Could you check a few things on this model? Use its own coordinates, in mm. A direction names the side the tool comes from. Give positions to 0.01 mm unless a question says otherwise; leave off trailing zeros. Loops run counter-clockwise (first coordinate to the right, second up) from the corner with the lowest first, then second, coordinate; pieces in that order, holes last. Notation, with made-up numbers: M -39,51 L -34,51 A27 cw -34,76 Z; hole C 41.25,44 d9. An arc over 180 degrees is marked long. Use a Markdown table: item, result. Add a question column.
1) Suppose I cut it at D-D on x = 8.5. List the corners of the cut face in (y, z) for me, and give its area (3 significant figures).
2) We'd pull the mould along Z, two halves only. Please class faces 3 (the flat face through (0, 0, -92.202)), 4 (the flat face through (0, 0, 0)), 5 (the cylindrical face through (1.323, 10.074, -70.11)): +Z half, -Z half, draft (parallel to the pull), parting line (faces both ways), or undercut.
3) If I drill on line 1 along Z through (x, y) = (7.25, 3.5); line 2 along Y through (x, z) = (-0.25, -9.5); line 3 along X through (y, z) = (2.5, -30.5), over which ranges is the centre line in solid material (lowest first)? Write a range as [from, to].
4) Which directions (+Z, -Z, +X, -X, +Y, -Y) give clear straight access to the entire face, cutting with the end or side of a thin tool? Please do faces 1 (the cylindrical face through (-1.38, -6.2, -29.8)), 2 (the flat face through (0, -7, -79.502)).
5) Suppose I cut it at C-C on z = -50. List the corners of the cut face in (x, y) for me.
6) Suppose I cut it at A-A on y = 0. List the corners of the cut face in (x, z) for me, and give its area (3 significant figures).
7) Will these pins go through, and if not, where does the flat tip stop? pin 1 Ø6 at (x, z) = (4, -66.5) entering from -Y; pin 2 Ø12 at (y, z) = (6, -56) entering from +X; pin 3 Ø8 at (y, z) = (-2.5, -40.5) entering from -X.
```python
from build123d import *

# Parameters (mm, degrees)
SKETCH1_R           = 6.35
BOSS_EXTRUDE1_DEPTH = 92.202
BOSS_EXTRUDE2_START = -12.7
SKETCH2_R           = 10.16
BOSS_EXTRUDE2_DEPTH = 19.05


with BuildPart() as part:
    # Sketch1 → Boss-Extrude1 (new body)
    with BuildSketch(Plane.XY):
        Circle(SKETCH1_R)
    extrude(amount=-BOSS_EXTRUDE1_DEPTH)

    # Sketch2 → Boss-Extrude2 (add)
    with BuildSketch(Plane(origin=(0, 0, -92.202), x_dir=(-1, 0, 0), z_dir=(0, 0, -1)).offset(BOSS_EXTRUDE2_START)):
        Circle(SKETCH2_R)
    extrude(amount=-BOSS_EXTRUDE2_DEPTH)


solid = part.part
```
Answer block:
| question | item | result |
|---|---|---|
| 1 | outline | M -5.57,-79.5 L 5.57,-79.5 L 5.57,-60.45 L -5.57,-60.45 Z |
| 1 | area | 212 mm^2 |
| 2 | face 3 | -Z half |
| 2 | face 4 | +Z half |
| 2 | face 5 | draft |
| 3 | line 1 | z = [-79.5, -60.45] |
| 3 | line 2 | y = [-6.35, 6.35] |
| 3 | line 3 | x = [-5.84, 5.84] |
| 4 | face 1 | +Z |
| 4 | face 2 | -Z |
| 5 | outline | C 0,0 d12.7 |
| 6 | outline | M -10.16,-79.5 L -6.35,-79.5 L -6.35,-92.2 L 6.35,-92.2 L 6.35,-79.5 L 10.16,-79.5 L 10.16,-60.45 L 6.35,-60.45 L 6.35,0 L -6.35,0 L -6.35,-60.45 L -10.16,-60.45 Z |
| 6 | area | 1,320 mm^2 |
| 7 | pin 1 | stops at y = -10.11 |
| 7 | pin 2 | stops at x = 9.97 |
| 7 | pin 3 | stops at x = -6.35 |
